Geometry check sheet. Reference: drawing and pictorial views, mm from the part's lowest x, y, z. A direction names the side the tool comes from. Coordinates: 2 decimals unless noted, no trailing zeros. Write each loop counter-clockwise with the first axis right and the second up, starting at its lowest first coordinate (ties: lowest second). Pieces come first, ordered by that corner, then holes. Notation, with made-up numbers: (2, 88.25) - (19, 88.25) arc R21 cw to (19, 108.25) - close; hole circle Ø2 at (76, 1). An arc over 180 degrees is marked (long way). Answer as a JSON object with one key per item and string values. Group by question number.
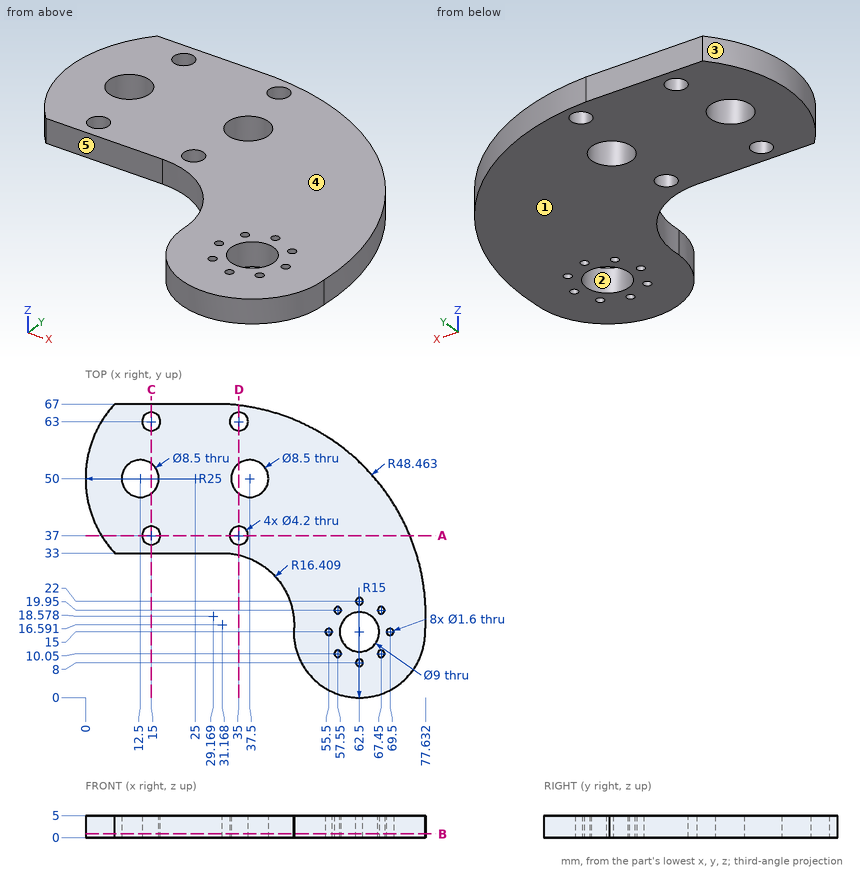
(1) Section check D-D (x = 35). Record the cut outline in (y, z).
(2) Material ranges on L1, parallel to Y at x = 15, z = 1.8 (1 decimal); L2, parallel to X at y = 47, z = 4.15 (1 decimal); L3, parallel to Y at x = 35, z = 1 (1 decimal), recorded low to high. Write a range as [from, to].
(3) Section check B-B (z = 0.85). Count the separate pieces of the cut face and the enclosed holes in it, and give its area (3 significant figures).
(4) Draft check along Y on the marked faces 1, 2 and 3. Enter one of: +Y half, -Y half, draft (parallel to the pull), parting line (faces both ways), or undercut.
(5) Gauge pin test, flat ends, axial feed: pin 1 (2.5 mm diameter, centred on x = 18, z = 2, fed in from -Y); pin 2 (3.5 mm diameter, centred on x = 35, y = 37, fed in from +Z); pin 3 (2 mm diameter, centred on y = 51.5, z = 2, fed in from +X) (1 decimal); pin 4 (3 mm diameter, centred on y = 57.5, z = 2.5, fed in from +X) (1 decimal). Record the tip position at first contact, or that the pin passes through.
(6) Set-up check for the marked faces 4 and 5: record each of +Z, -Z, +X, -X, +Y, -Y from which the full face is reachable in a straight line by a thin tool's end or side.
(7) Section check A-A (y = 37). Record the cut outline in (x, z) (1 decimal).
(8) Section check C-C (x = 15). Record the cut outline in (y, z).
Conclusion:
{
 "1": {"outline": "(32.55, 0) - (34.9, 0) - (34.9, 5) - (32.55, 5) - close; (39.1, 0) - (46.56, 0) - (46.56, 5) - (39.1, 5) - close; (53.44, 0) - (60.9, 0) - (60.9, 5) - (53.44, 5) - close; (65.1, 0) - (66.69, 0) - (66.69, 5) - (65.1, 5) - close"},
 "2": {"L1": "y = [33, 34.9], [39.1, 46.6], [53.4, 60.9], [65.1, 67]", "L2": "x = [0.2, 9.5], [15.5, 34.5], [40.5, 68.4]", "L3": "y = [32.5, 34.9], [39.1, 46.6], [53.4, 60.9], [65.1, 66.7]"},
 "3": {"separate pieces": "1", "enclosed holes": "15", "area": "2,770 mm^2"},
 "4": {"face 1": "draft", "face 2": "undercut", "face 3": "parting line"},
 "5": {"pin 1": "stops at y = 33", "pin 2": "passes through", "pin 3": "stops at x = 65.6", "pin 4": "stops at x = 60"},
 "6": {"face 4": "+Z, +X, -X, +Y, -Y", "face 5": "+Z, -Z, -X, -Y"},
 "7": {"outline": "(3.6, 0) - (12.9, 0) - (12.9, 5) - (3.6, 5) - close; (17.1, 0) - (32.9, 0) - (32.9, 5) - (17.1, 5) - close; (37.1, 0) - (74, 0) - (74, 5) - (37.1, 5) - close"},
 "8": {"outline": "(33, 0) - (34.9, 0) - (34.9, 5) - (33, 5) - close; (39.1, 0) - (46.56, 0) - (46.56, 5) - (39.1, 5) - close; (53.44, 0) - (60.9, 0) - (60.9, 5) - (53.44, 5) - close; (65.1, 0) - (67, 0) - (67, 5) - (65.1, 5) - close"}
}
